CAD build for the part. Positions are in the model's coordinates, mm. Face numbers are marked on the shaded views. A direction names the side the tool comes from. Coordinates: 2 decimals unless noted, no trailing zeros. Write each loop counter-clockwise with the first axis right and the second up, starting at its lowest first coordinate (ties: lowest second). Pieces come first, ordered by that corner, then holes. Notation, with made-up numbers: (25.5, 54.5) -> (63.5, 54.5) arc R16 cw to (63.5, 83.5) -> close; hole circle Ø2 at (36.5, 49). An arc over 180 degrees is marked (long way). Answer as CSV lines item,"result".
```python
from build123d import *

# Parameters (mm, degrees)
EXTRUDE_3_DEPTH          = 8
SKETCH_4_W               = 50
SKETCH_4_H               = 40
EXTRUDE_4_DEPTH          = 2
FILLET_1_R               = 2
CUT_EXTRUDE_1_DEPTH      = 3
CUT_EXTRUDE_2_DEPTH      = 44.350317185
CUT_EXTRUDE_2_DEPTH_BACK = 44.350317185
SKETCH_3_4_R             = 1.6
SKETCH_6_W               = 9
SKETCH_6_H               = 9
CUT_EXTRUDE_3_DEPTH      = 2
FILLET_3_R               = 2
EXTRUDE_5_DEPTH          = 16


with BuildPart() as part:
    # Эскиз3 → Бобышка-Вытянуть3 (new body)
    with BuildSketch(Plane.XY):
        with BuildLine():
            ThreePointArc((-21.292484919, 9.830060324), (-21.212678125, 0.149287499), (-16.586602566, 8.653589736))
            Line((-16.586602566, 8.653589736), (-15.5, 13))
            Line((-15.5, 13), (-20.5, 13))
            Line((-20.5, 13), (-21.292484919, 9.830060324))
        make_face()
    extrude(amount=EXTRUDE_3_DEPTH)

    # Эскиз4 → Бобышка-Вытянуть4 (add)
    with BuildSketch(Plane(origin=(0, 13, 0), x_dir=(1, 0, 0), z_dir=(0, 1, 0))):
        with Locations((-4.5, -8)):
            Rectangle(SKETCH_4_W, SKETCH_4_H)
    extrude(amount=EXTRUDE_4_DEPTH)

    # Скругление1
    fillet_1_edges = [part.edges().sort_by_distance(p)[0] for p in [
        (-29.5, 14, -12),
        (-29.5, 14, 28),
        (20.5, 14, 28),
        (20.5, 14, -12),
    ]]
    fillet(fillet_1_edges, radius=FILLET_1_R)

    # Эскиз3<3> → Вырез-Вытянуть1 (cut)
    with BuildSketch(Plane.XY):
        Polygon((-21.625, 7.814582562), (-23.25, 5), (-21.625, 2.185417438), (-18.375, 2.185417438), (-16.75, 5), (-18.375, 7.814582562), align=None)
    extrude(amount=CUT_EXTRUDE_1_DEPTH, mode=Mode.SUBTRACT)

    # Эскиз3<4> → Вырез-Вытянуть2 (cut, two sides: drawn at the far end of the back side and taken through both)
    with BuildSketch(Plane.XY.offset(-CUT_EXTRUDE_2_DEPTH_BACK)):
        with Locations((-20, 5)):
            Circle(SKETCH_3_4_R)
    extrude(amount=CUT_EXTRUDE_2_DEPTH + CUT_EXTRUDE_2_DEPTH_BACK, mode=Mode.SUBTRACT)

    # Эскиз6 → Вырез-Вытянуть3 (cut)
    with BuildSketch(Plane(origin=(0, 15, 0), x_dir=(1, 0, 0), z_dir=(0, 1, 0))):
        with Locations((-25, -8)):
            Rectangle(SKETCH_6_W, SKETCH_6_H)
    extrude(amount=-CUT_EXTRUDE_3_DEPTH, mode=Mode.SUBTRACT)

    # Скругление3
    fillet_3_edges = [part.edges().sort_by_distance(p)[0] for p in [
        (-29.5, 14, 12.5),
        (-29.5, 14, 3.5),
        (-20.5, 14, 3.5),
        (-20.5, 14, 12.5),
    ]]
    fillet(fillet_3_edges, radius=FILLET_3_R)

    # Эскиз3<5> → Бобышка-Вытянуть5 (add)
    with BuildSketch(Plane.XY):
        with BuildLine():
            ThreePointArc((-21.292484919, 9.830060324), (-18.787321875, 9.850712501), (-16.586602566, 8.653589736))
            Line((-16.586602566, 8.653589736), (-15.5, 13))
            Line((-15.5, 13), (-20.5, 13))
            Line((-20.5, 13), (-21.292484919, 9.830060324))
        make_face()
    extrude(amount=EXTRUDE_5_DEPTH)


solid = part.part
```
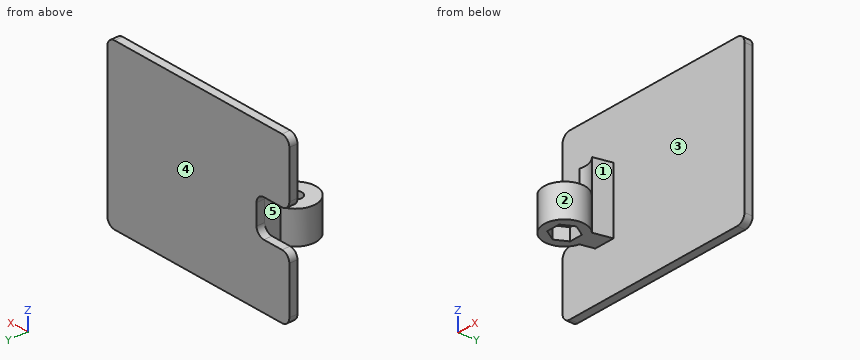
Item 1: Two-plate mould, pull along X, no slides. Class the marked faces 1, 2 and 3: pulls with the +X half, pulls with the -X half, needs draft (parallel to the pull), parting line crosses it, or undercut.
Answer below:
face 1,"pulls with the +X half"
face 2,"parting line crosses it"
face 3,"needs draft"
Item 2: Saw through at B-B on z = -7. Give the cut face in (x, y), and give its area (3 significant figures).
Answer below:
outline,"(-29.5, 13) -> (20.5, 13) -> (20.5, 15) -> (-29.5, 15) -> close"
area,"100 mm2"
Item 3: Flat gauge pins, fed straight in: pin 1 (1.7 mm diameter, centred on x = -20.5, y = 4, fed in from -Z); pin 2 (20 mm diameter, centred on x = -11.5, z = 13.5, fed in from -Y); pin 3 (2 mm diameter, centred on x = -17, y = 11.5, fed in from +Z). Where does each tip first touch, or does it go through?
Answer below:
pin 1,"stops at z = 3"
pin 2,"stops at y = 0"
pin 3,"stops at z = 16"
Item 4: Wall check: line 1 (X direction, y = 5, z = 6.4); line 2 (Y direction, x = -20, z = 4.35); line 3 (Y direction, x = 17, z = 7). Give the ranges that are in metal, low to high. Write a range as from..to.
Answer below:
line 1,"x = -25..-21.6, -18.4..-15"
line 2,"y = 0..3.4, 6.6..15"
line 3,"y = 13..15"
Item 5: 3-axis set-ups, long thin cutter, end or side, ignore diameter. For the marked faces 4 and 5: which of +Z, -Z, +X, -X, +Y, -Y reach the whole face in a straight line?
Answer below:
face 4,"+Z, -Z, +X, -X, +Y"
face 5,"+Z, -Z, -X"
Item 6: Saw through at A-A on y = 13.75. Give the cut face in (x, z).
Answer below:
outline,"(-29.5, -10) arc R2 ccw to (-27.5, -12) -> (18.5, -12) arc R2 ccw to (20.5, -10) -> (20.5, 26) arc R2 ccw to (18.5, 28) -> (-27.5, 28) arc R2 ccw to (-29.5, 26) -> (-29.5, 14.5) arc R2 ccw to (-27.5, 12.5) -> (-22.5, 12.5) arc R2 cw to (-20.5, 10.5) -> (-20.5, 5.5) arc R2 cw to (-22.5, 3.5) -> (-27.5, 3.5) arc R2 ccw to (-29.5, 1.5) -> close"
Item 7: Saw through at C-C on x = -13. Give the cut face in (y, z), and give its area (3 significant figures).
Answer below:
outline,"(13, -12) -> (15, -12) -> (15, 28) -> (13, 28) -> close"
area,"80.0 mm2"
